For this review, use the dimensioned drawing (mm, ordinates from the lowest corner) and the shaded views. A direction names the side the tool comes from. Give positions to 0.01 mm unless a question says otherwise; leave off trailing zeros. Write each loop counter-clockwise with the first axis right and the second up, starting at its lowest first coordinate (ties: lowest second). Pieces come first, ordered by that corner, then holes. Notation, with made-up numbers: M 61,37 L 110,37 A17 ccw 110,45 Z; hole C 17.5,84 d4. An arc over 180 degrees is marked long. One line per item, written item: value. Start each with the question number.
Item 1: Consider section A-A, the plane z = 5.5. Write out the cut boundary in (x, y), and give its area (3 significant figures).
Item 2: To check wall thickness, follow probe 1 along X at (y, z) = (10.5, 1.75); probe 2 along Y at (x, z) = (3, 0.5); probe 3 along X at (y, z) = (14.5, 7.5). State the ranges of each line that lie inside material, in increasing order.
Item 3: Consider section D-D, the plane z = 6.75. Write out the cut boundary in (x, y).
Item 4: Consider section C-C, the plane y = 14.25. Write out the cut boundary in (x, z).
Item 5: Tool access review of the marked faces 1, 2 and 3: name each direction out of +Z, -Z, +X, -X, +Y, -Y from which nothing blocks a thin tool from reaching the whole face with its end or side.
Item 6: Clearance check with flat-ended pins moving along their axes: pin 1 Ø2 at (x, y) = (6.5, 16.5) entering from +Z; pin 2 Ø2 at (x, z) = (6, 0.5) entering from +Y; pin 3 Ø1 at (y, z) = (6, 0.5) entering from -X. State where each tip first meets the part, or that it passes through.
Item 7: Mouldability with a two-part tool opening along X and no side actions: class the marked faces 4, 5 and 6 as released by +X, released by -X, zero draft, split by the parting line, or undercut.
Item 8: Consider section B-B, the plane x = 5. Write out the cut boundary in (y, z).
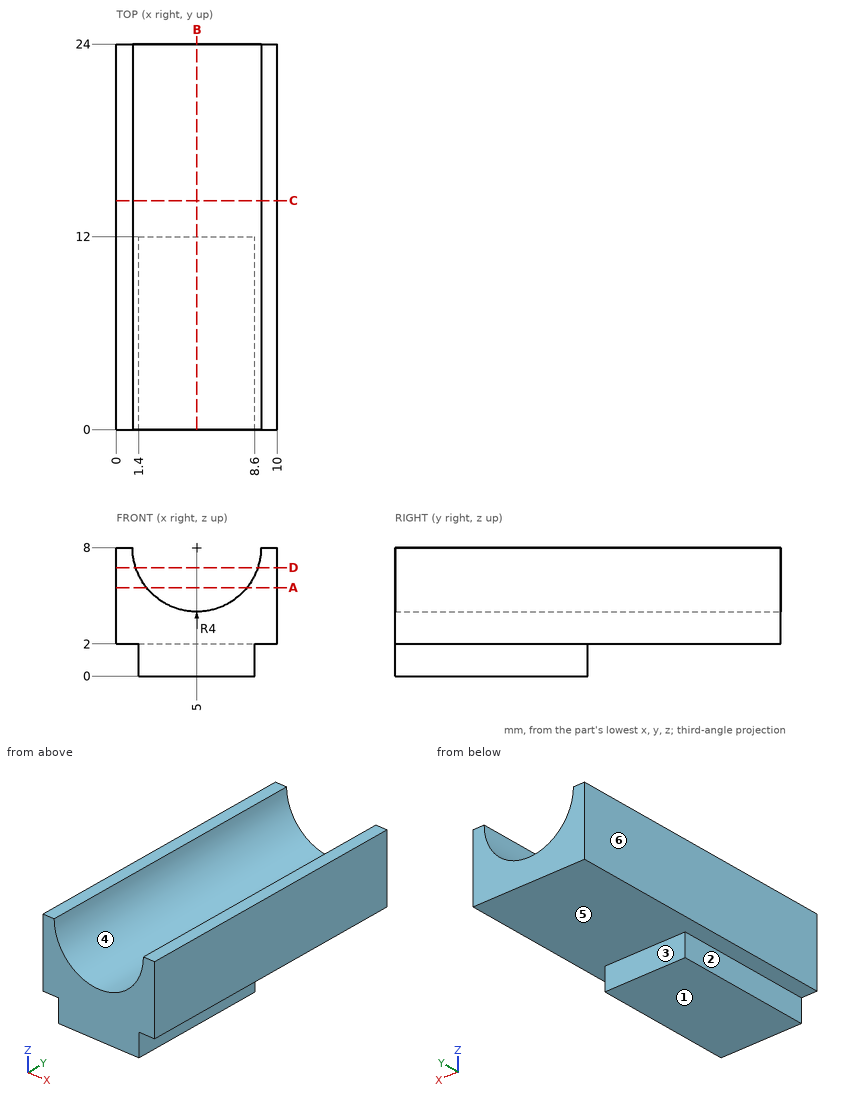
Model answer:
1. outline: M 0,0 L 1.88,0 L 1.88,24 L 0,24 Z; M 8.12,0 L 10,0 L 10,24 L 8.12,24 Z
1. area: 90.1 mm2
2. probe 1: x = 1.4 to 8.6
2. probe 2: y = 0 to 12
2. probe 3: x = 0 to 1.03, 8.97 to 10
3. outline: M 0,0 L 1.2,0 L 1.2,24 L 0,24 Z; M 8.8,0 L 10,0 L 10,24 L 8.8,24 Z
4. outline: M 0,2 L 10,2 L 10,8 L 9,8 A4 cw 1,8 L 0,8 Z
5. face 1: -Z, +X, -X, +Y, -Y
5. face 2: -Z, -X, +Y, -Y
5. face 3: -Z, +X, -X, +Y
6. pin 1: stops at z = 4.88
6. pin 2: stops at y = 12
6. pin 3: stops at x = 1.4
7. face 4: undercut
7. face 5: zero draft
7. face 6: released by -X
8. outline: M 0,0 L 12,0 L 12,2 L 24,2 L 24,4 L 0,4 Z
